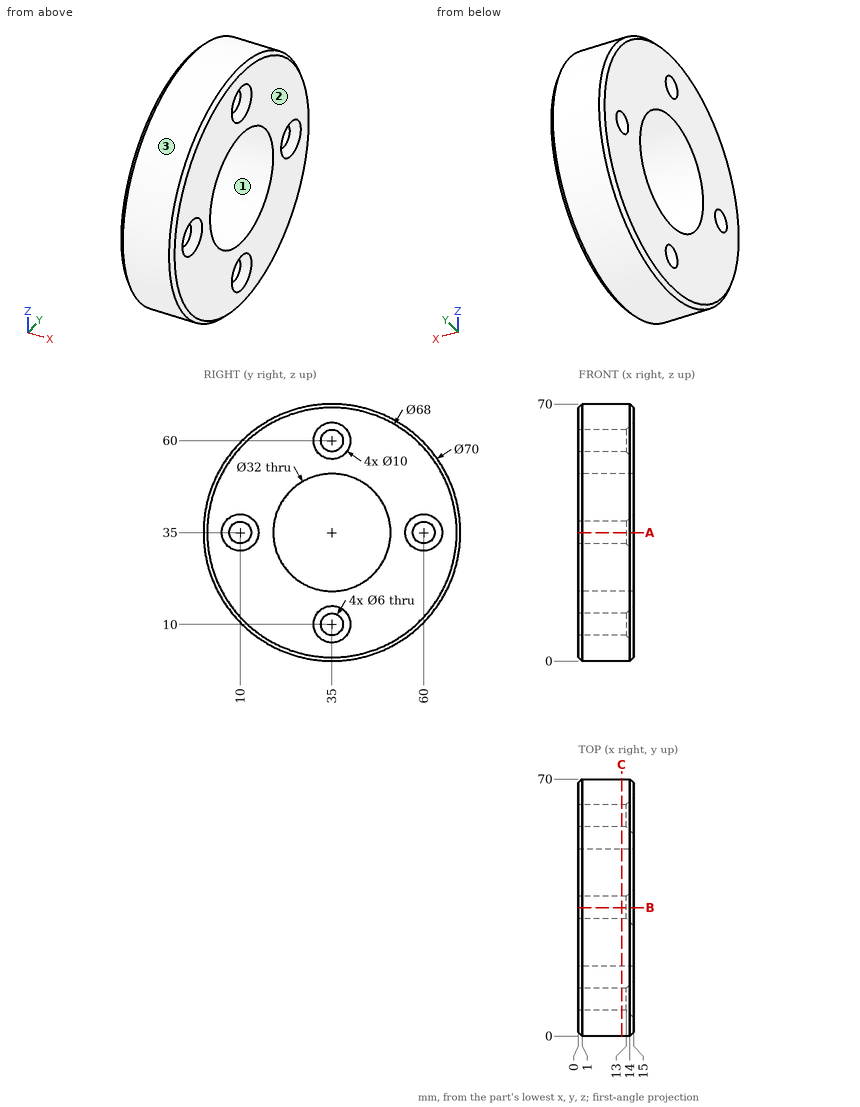
Geometry: see drawing. Coordinates: mm, zero at the bounding-box minimum. Round coordinates to 2 decimals unless told otherwise and drop trailing zeros. Write each loop counter-clockwise with the first axis right and the second up, starting at its lowest first coordinate (ties: lowest second). Pieces come first, ordered by that corner, then holes. Notation, with made-up numbers: (-29.75, 39) - (-15.75, 39) arc R17 ccw to (-15.75, 50) - close; hole circle Ø8 at (-11, 44). An arc over 180 degrees is marked (long way). Use CSV: the item, a comma, the result in double quotes. Start each with the question number.
(1) Cut plane A-A, the plane z = 35. Return loops of the section in (x, y), and give its area (3 significant figures).
(2) Mould query, pull axis Y, two halves, no side actions, for the marked faces 1, 2 and 3. Classes: pulls with the +Y half, pulls with the -Y half, needs draft (parallel to the pull), parting line crosses it, or undercut.
(3) Material intervals for probe 1 along Z at (x, y) = (7.25, 35); probe 2 along Z at (x, y) = (8.75, 37); probe 3 along Y at (x, z) = (5, 10), sorted ascending. Write a range as [from, to].
(4) Cut plane C-C, the plane x = 11.75. Return loops of the section in (y, z).
(5) First-contact query: pin 1 Ø8 at (y, z) = (35, 10) entering from -X; pin 2 Ø1 at (x, y) = (3.5, 36) entering from -Z; pin 3 Ø2 at (x, z) = (4.5, 28) entering from +Y; pin 4 Ø2 at (x, y) = (2.5, 12.5) entering from +Z. Flat tips, straight axial feed; report the tip coordinate or a pass-through.
Geometry says:
1,outline,"(0, 1) - (1, 0) - (14, 0) - (15, 1) - (15, 5) - (13, 7) - (0, 7) - close; (0, 13) - (13, 13) - (15, 15) - (15, 19) - (0, 19) - close; (0, 51) - (15, 51) - (15, 55) - (13, 57) - (0, 57) - close; (0, 63) - (13, 63) - (15, 65) - (15, 69) - (14, 70) - (1, 70) - (0, 69) - close"
1,area,"380 mm²"
2,face 1,"undercut"
2,face 2,"needs draft"
2,face 3,"parting line crosses it"
3,probe 1,"[0, 7], [13, 19], [51, 57], [63, 70]"
3,probe 2,"[0.06, 7.76], [12.24, 19.13], [50.87, 57.76], [62.24, 69.94]"
3,probe 3,"[10.51, 32], [38, 59.49]"
4,outline,"circle Ø70 at (35, 35); hole circle Ø6 at (10, 35); hole circle Ø32 at (35, 35); hole circle Ø6 at (35, 10); hole circle Ø6 at (35, 60); hole circle Ø6 at (60, 35)"
5,pin 1,"x = 0"
5,pin 2,"z = 0"
5,pin 3,"y = 69.48"
5,pin 4,"z = 62.62"
